Design review of the part built by this model. Coordinates are the model's own, in mm. Face numbers are marked on the shaded views. A direction names the side the tool comes from. Coordinates: 2 decimals unless noted, no trailing zeros. Write each loop counter-clockwise with the first axis right and the second up, starting at its lowest first coordinate (ties: lowest second). Pieces come first, ordered by that corner, then holes.
Q1. To check wall thickness, follow probe 1 along X at (y, z) = (-30.5, 18.5); probe 2 along Y at (x, z) = (21.5, 19); probe 3 along Z at (x, y) = (-6, -39). State the ranges of each line that lie inside material, in increasing order.
Q2. Add section C-C, the plane y = -28. Give the boundary of the cut face in (x, z).
Q3. Add section B-B, the plane x = 9. Give the boundary of the cut face in (y, z), plus the area to 3 significant figures.
Q4. The part is to be moulded in two halves that separate along X. For the marked faces 1, 2 and 3, say which applies: +X half, -X half, draft (parallel to the pull), parting line (faces both ways), or undercut.
Q5. Clearance check with flat-ended pins moving along their axes: pin 1 Ø2 at (x, y) = (-47.5, 41) entering from +Z; pin 2 Ø10 at (x, y) = (-31, -30.5) entering from -Z; pin 3 Ø6 at (y, z) = (19, 75) entering from +X. State where each tip first meets the part, or that it passes through.
Q6. Add section A-A, the plane z = 18.5. Give the boundary of the cut face in (x, y), plus the area to 3 significant figures.
Q7. Machinability: for the marked faces 4 and 5, which of the approach directions +Z, -Z, +X, -X, +Y, -Y give a long, thin tool a straight path to every point of the face, cutting with its end or side? Answer none if there is none.
Q8. Add section D-D, the plane z = 51.5. Give the boundary of the cut face in (x, y), plus the area to 3 significant figures.
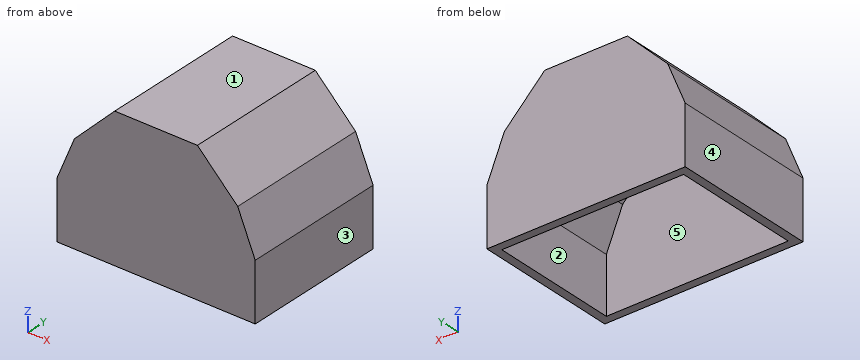
from build123d import *

# Parameters (mm, degrees)
F0_W     = 152.5266170502
F0_H     = 112.4007552862
F1_DEPTH = 107.95
F2_SIZE  = 44.45
F3_SIZE  = 44.45
F4_SIZE  = 19.05
F5_SIZE  = 19.05
F6_T     = -6.35


with BuildPart() as f1:
    # F0 (on Top) → F1 (new body)
    with BuildSketch(Plane.XY):
        Rectangle(F0_W, F0_H)
    extrude(amount=F1_DEPTH)

    # F2
    f2_edges = [f1.edges().sort_by_distance(p)[0] for p in [
        (-76.263309, 0, 107.95),
    ]]
    chamfer(f2_edges, length=F2_SIZE)

    # F3
    f3_edges = [f1.edges().sort_by_distance(p)[0] for p in [
        (76.263309, 0, 107.95),
    ]]
    chamfer(f3_edges, length=F3_SIZE)

    # F4
    f4_edges = [f1.edges().sort_by_distance(p)[0] for p in [
        (-76.263309, 0, 63.5),
    ]]
    chamfer(f4_edges, length=F4_SIZE)

    # F5
    f5_edges = [f1.edges().sort_by_distance(p)[0] for p in [
        (76.263309, 0, 63.5),
    ]]
    chamfer(f5_edges, length=F5_SIZE)

    # F6
    f6_openings = [f1.faces().sort_by_distance(p)[0] for p in [
        (0, 0, 0),
    ]]
    offset(amount=F6_T, openings=f6_openings)


solid = f1.part
Here are the results:
1. probe 1: x = -76.26 to -69.91, 69.91 to 76.26
1. probe 2: y = -56.2 to -49.85, 49.85 to 56.2
1. probe 3: z = 101.6 to 107.95
2. outline: (-76.26, 0) - (-69.91, 0) - (-69.91, 43.19) - (-57.41, 73.37) - (-29.18, 101.6) - (29.18, 101.6) - (57.41, 73.37) - (69.91, 43.19) - (69.91, 0) - (76.26, 0) - (76.26, 44.45) - (62.79, 76.97) - (31.81, 107.95) - (-31.81, 107.95) - (-62.79, 76.97) - (-76.26, 44.45) - close
3. outline: (-56.2, 0) - (-49.85, 0) - (-49.85, 101.6) - (49.85, 101.6) - (49.85, 0) - (56.2, 0) - (56.2, 107.95) - (-56.2, 107.95) - close
3. area: 2,000 mm2
4. face 1: draft
4. face 2: undercut
4. face 3: +X half
5. pin 1: stops at z = 93.26
5. pin 2: stops at z = 94.78
5. pin 3: stops at x = 64.85
6. outline: (-76.26, -56.2) - (76.26, -56.2) - (76.26, 56.2) - (-76.26, 56.2) - close; hole (-69.91, -49.85) - (69.91, -49.85) - (69.91, 49.85) - (-69.91, 49.85) - close
6. area: 3,200 mm2
7. face 4: +Z, -Z, -X, +Y, -Y
7. face 5: -Z
8. outline: (-73.34, -56.2) - (73.34, -56.2) - (73.34, 56.2) - (-73.34, 56.2) - close; hole (-66.47, -49.85) - (66.47, -49.85) - (66.47, 49.85) - (-66.47, 49.85) - close
8. area: 3,230 mm2
